Here's the drawing with two shaded views (mm, measured from the low corner). I have some questions. A direction names the side the tool comes from. Round coordinates to 2 decimals unless told otherwise and drop trailing zeros. Write each loop counter-clockwise with the first axis right and the second up, starting at its lowest first coordinate (ties: lowest second). Pieces come first, ordered by that corner, then holes. Notation, with made-up numbers: M 37,41.5 L 92,41.5 A31 cw 92,70.5 Z; hole C -35,76 d8. An arc over 180 degrees is marked long. Answer as a JSON object with one key per item and string values. Group by question number.
1) Please list where these lines run through material, in increasing order: L1, parallel to Z at x = 22, y = 24 (3 decimals); L2, parallel to X at y = 18, z = 74; L3, parallel to X at y = 23, z = 95. Write a range as [from, to].
2) I'm going to push flat-ended pins straight in: pin 1 Ø2 at (x, z) = (24.5, 119) entering from -Y; pin 2 Ø12 at (y, z) = (37.5, 34) entering from -X; pin 3 Ø5 at (y, z) = (50, 46.5) entering from -X. Where does each tip first touch, or does it pass through?
3) If we mould it in two halves opening along X, with no side actions, what happens to the marked faces 1, 2 and 3? For each: +X half, -X half, draft (parallel to the pull), parting line (faces both ways), or undercut.
4) Suppose I cut it at A-A, the plane y = 20.5. Write out the boundary of the cut face in (x, z) (3 decimals), and give its area (3 significant figures).
5) Suppose I cut it at B-B, the plane z = 89.5. Write out the boundary of the cut face in (x, y) (3 decimals).
6) Suppose I cut it at C-C, the plane x = 57.15. Write out the boundary of the cut face in (y, z) (3 decimals).
7) On a 3-axis mill with a long thin cutter (end or side, diameter ignored), from which of +Z, -Z, +X, -X, +Y, -Y can I reach the whole of each face in a straight line? I mean the marked faces 4 and 5. Say none if no direction works.
8) Suppose I cut it at D-D, the plane y = 9.5. Write out the boundary of the cut face in (x, z) (3 decimals), and give its area (3 significant figures).
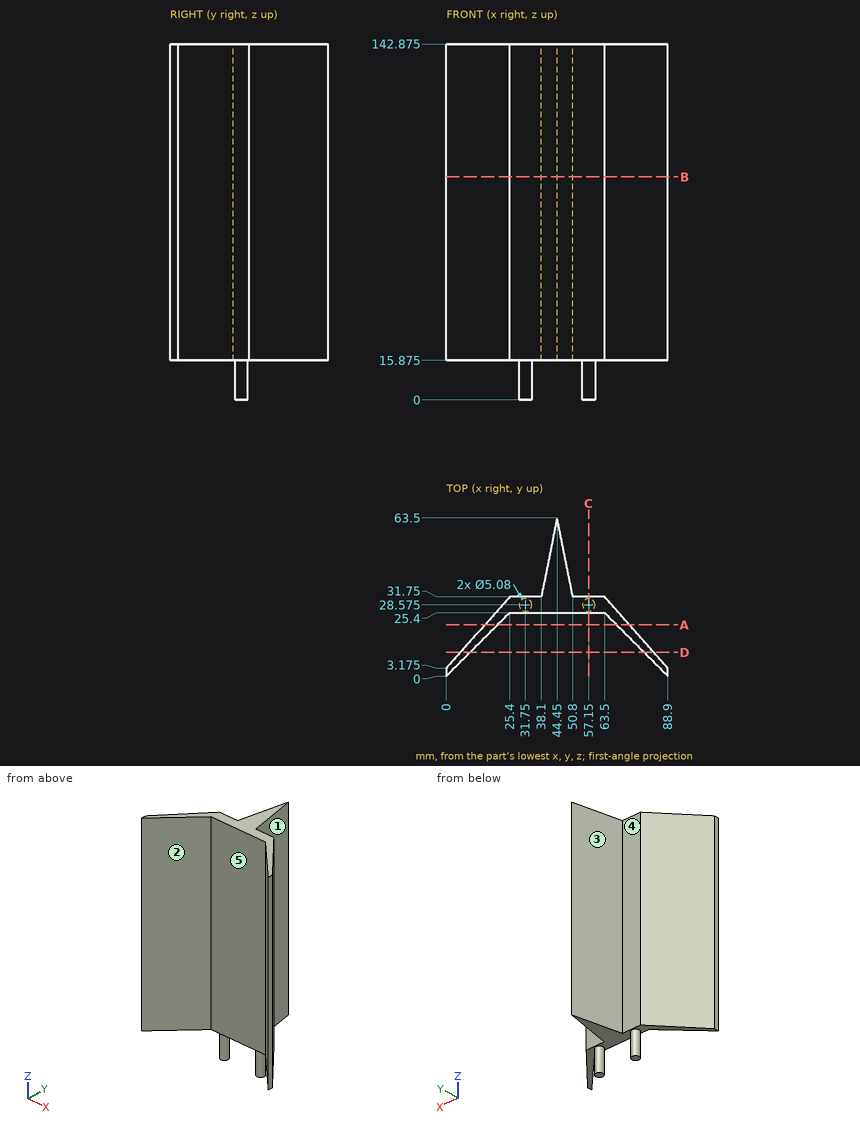
Results:
{
 "1": {"L1": "[15.875, 142.875]", "L2": "[13.18, 18], [70.9, 75.72]", "L3": "[17.62, 23], [65.9, 71.28]"},
 "2": {"pin 1": "y = 23.5", "pin 2": "x = 25.18", "pin 3": "x = 41.25"},
 "3": {"face 1": "+X half", "face 2": "undercut", "face 3": "-X half"},
 "4": {"outline": "M 15.4,15.875 L 20.5,15.875 L 20.5,142.875 L 15.4,142.875 Z; M 68.4,15.875 L 73.5,15.875 L 73.5,142.875 L 68.4,142.875 Z", "area": "1,300 mm^2"},
 "5": {"outline": "M 0,0 L 25.4,25.4 L 63.5,25.4 L 88.9,0 L 88.9,3.175 L 63.5,31.75 L 50.8,31.75 L 44.45,63.5 L 38.1,31.75 L 25.4,31.75 L 0,3.175 Z"},
 "6": {"outline": "M 25.4,15.875 L 26.035,15.875 L 26.035,0 L 31.115,0 L 31.115,15.875 L 31.75,15.875 L 31.75,142.875 L 25.4,142.875 Z"},
 "7": {"face 4": "+Z, -Z, -X, +Y", "face 5": "+Z, -Z, -Y"},
 "8": {"outline": "M 5.622,15.875 L 9.5,15.875 L 9.5,142.875 L 5.622,142.875 Z; M 79.4,15.875 L 83.278,15.875 L 83.278,142.875 L 79.4,142.875 Z", "area": "985 mm^2"}
}
